Input: dimensioned drawing with shaded views. Units: mm. Origin: part minimum x, y, z. A direction names the side the tool comes from. Give positions to 0.01 mm unless a question says otherwise; leave off trailing zeros. Loops run counter-clockwise (first coordinate to the right, second up) from the corner with the lowest first, then second, coordinate; pieces in that order, holes last. Notation, with made-up numbers: (-20, -29.75) -> (-9, -29.75) arc R23 ccw to (-9, -16.75) -> close; hole circle Ø9 at (-6.75, 53). An arc over 180 degrees is marked (long way). Answer in a Markdown table with one row per item. Add a question column.
1) Line query: line 1 (Y direction, x = 41, z = 23.5); line 2 (X direction, y = 44, z = 18). Output: solid intervals per line, ascending. Write a range as from..to.
2) Access query for the marked faces 1, 2, 3 and 4. Directions: +Z, -Z, +X, -X, +Y, -Y. A direction counts if a zero-diameter tool reaches every point of the face in a straight line with its end or side. Return the directions, or none.
3) First-contact query: P1, Ø5, axis at x = 6, z = 19.5, coming from the -Y side; P2, Ø5, axis at y = 45, z = 13.5, coming from the +X side; P3, Ø8, axis at y = 47, z = 26, coming from the -X side. Flat tips, straight axial feed; report the tip coordinate or a pass-through.
4) Section query B-B (y = 3). Return the cut outline in (x, z), plus the area to 3 significant figures.
5) Section query A-A (z = 22). Return the cut outline in (x, y), plus the area to 4 significant figures.
6) Section query C-C (x = 42). Return the cut outline in (y, z).
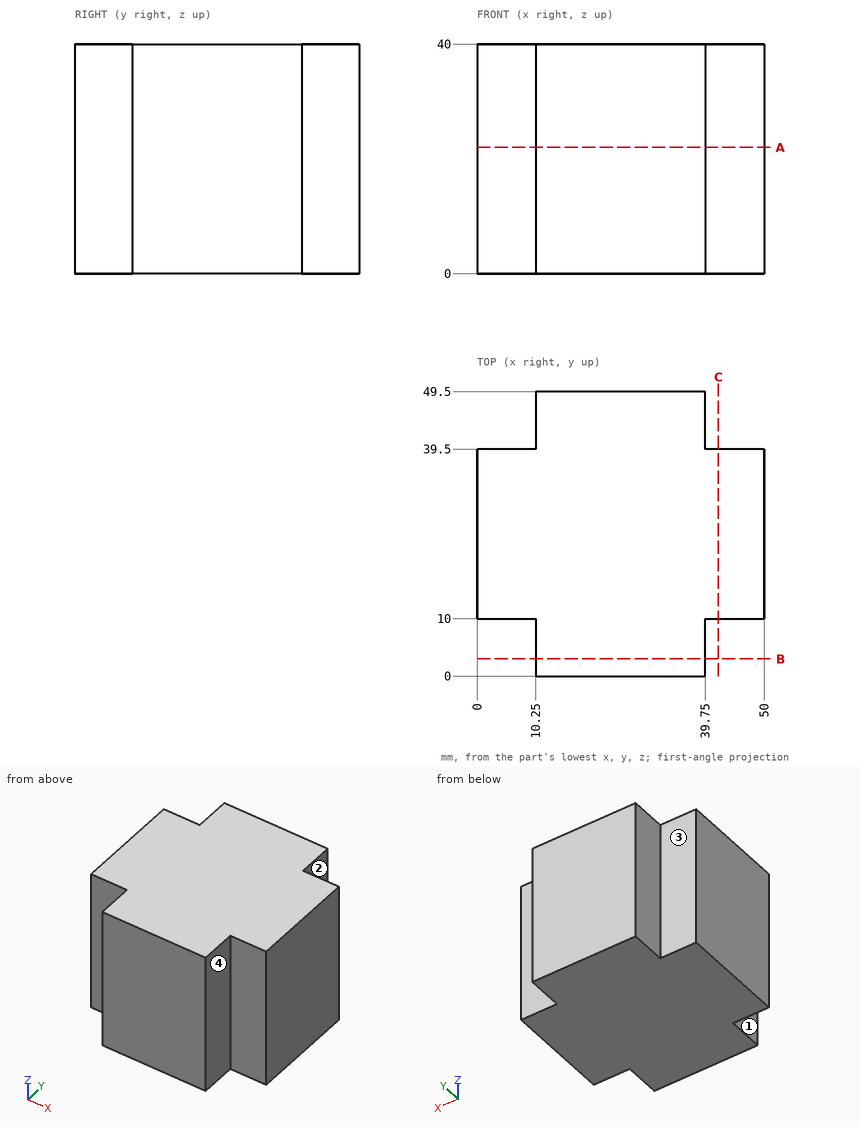
Evaluation:
| question | item | result |
|---|---|---|
| 1 | line 1 | 10..39.5 |
| 1 | line 2 | 10.25..39.75 |
| 2 | face 1 | +Z, -Z, -X, -Y |
| 2 | face 2 | +Z, -Z, +X, +Y |
| 2 | face 3 | +Z, -Z, -X, +Y |
| 2 | face 4 | +Z, -Z, +X, -Y |
| 3 | P1 | y = 10 |
| 3 | P2 | x = 39.75 |
| 3 | P3 | x = 10.25 |
| 4 | outline | (10.25, 0) -> (39.75, 0) -> (39.75, 40) -> (10.25, 40) -> close |
| 4 | area | 1,180 mm² |
| 5 | outline | (0, 10) -> (10.25, 10) -> (10.25, 0) -> (39.75, 0) -> (39.75, 10) -> (50, 10) -> (50, 39.5) -> (39.75, 39.5) -> (39.75, 49.5) -> (10.25, 49.5) -> (10.25, 39.5) -> (0, 39.5) -> close |
| 5 | area | 2,065 mm² |
| 6 | outline | (10, 0) -> (39.5, 0) -> (39.5, 40) -> (10, 40) -> close |
